Geometry: final body of the model. Coordinates: model frame, mm. Face numbers are marked on the shaded views. A direction names the side the tool comes from. Give positions to 0.01 mm unless a question says otherwise; leave off trailing zeros. Write each loop counter-clockwise with the first axis right and the second up, starting at its lowest first coordinate (ties: lowest second). Pieces come first, ordered by that corner, then holes. Notation, with made-up numbers: M -2,26.5 L 24,26.5 A29 ccw 24,49.5 Z; hole C -28,27 d7. An arc over 180 degrees is marked long. Use a Markdown table: item, result. Add a question column.
(1) Cut plane B-B (z = 21). Output: boundary loops of the cut face in (x, y).
(2) Draft query along Z for the marked faces 1, 2 and 3. Return one class per face: released by +Z, released by -Z, zero draft, split by the parting line, or undercut.
(3) Reachability of the marked faces 4 and 5 from +Z, -Z, +X, -X, +Y, -Y: full face, straight path, thin tool, end or side. Return the list, or none.
(4) Material intervals for L1, parallel to Z at x = 55.5, y = 70.5; L2, parallel to Z at x = 16.5, y = 74.5; L3, parallel to X at y = 66, z = 13.5, sorted ascending.
(5) Cut plane A-A (x = 50.5). Output: boundary loops of the cut face in (y, z).
(6) Pin query (flat end, axial travel): pin 1 Ø4 at (x, z) = (128.5, -13.5) entering from -Y; pin 2 Ø5 at (y, z) = (70, 12.5) entering from +X; pin 3 Ø1.6 at (y, z) = (72.5, -22) entering from -X; pin 4 Ø2 at (y, z) = (67.5, 26) entering from -X. Return the tip coordinate at first contact, or that it passes through.
```python
from build123d import *

# Parameters (mm, degrees)
BOX001002001_W                     = 70
BOX001002001_H                     = 15
BOX001002001_DEPTH                 = 2
BOX001002001002_W                  = 60
BOX001002001002_H                  = 15
BOX001002001002_DEPTH              = 2
BOX001002001002_PLACEMENT_ANGLE    = 209.99999
BOX001002001001_W                  = 60
BOX001002001001_H                  = 15
BOX001002001001_DEPTH              = 2
BOX001002001001_PITCH_ANGLE        = -31.999951
BOX001002001003_W                  = 26
BOX001002001003_H                  = 15
BOX001002001003_DEPTH              = 2
BOX001002001003_PLACEMENT_ANGLE    = 60.000023
BOX001002001003001_W               = 26
BOX001002001003001_H               = 15
BOX001002001003001_DEPTH           = 2
BOX001002001003001_PLACEMENT_ANGLE = 119.999977
BOX001002_W                        = 145
BOX001002_H                        = 15
BOX001002_DEPTH                    = 2


with BuildPart() as box001002001:
    # Box001002001 → Box001002001 (new body)
    with BuildSketch(Plane(origin=(49, -20, -23), x_dir=(1, 0, 0), z_dir=(0, 0, 1))):
        with Locations((35, 7.5)):
            Rectangle(BOX001002001_W, BOX001002001_H)
    extrude(amount=BOX001002001_DEPTH)


with BuildPart() as box001002001002:
    # Box001002001002 → Box001002001002 (new body)
    with BuildSketch(Plane.XY):
        with Locations((30, 7.5)):
            Rectangle(BOX001002001002_W, BOX001002001002_H)
    extrude(amount=BOX001002001002_DEPTH)


with BuildPart() as box001002001002_1:
    # Box001002001002 placement: moved
    add(box001002001002.part.moved(Location((49, -20, -21))).rotate(Axis((49, -20, -21), (0, 1, 0)), BOX001002001002_PLACEMENT_ANGLE))


with BuildPart() as box001002001001:
    # Box001002001001 → Box001002001001 (new body)
    with BuildSketch(Plane.XY):
        with Locations((30, 7.5)):
            Rectangle(BOX001002001001_W, BOX001002001001_H)
    extrude(amount=BOX001002001001_DEPTH)


with BuildPart() as box001002001001_1:
    # Box001002001001 pitch: moved
    add(box001002001001.part.rotate(Axis((0, 0, 0), (0, 1, 0)), BOX001002001001_PITCH_ANGLE))


with BuildPart() as box001002001001_2:
    # Box001002001001 placement: moved
    add(box001002001001_1.part.moved(Location((119, -20, -23))))


with BuildPart() as box001002001003:
    # Box001002001003 → Box001002001003 (new body)
    with BuildSketch(Plane.XY):
        with Locations((13, 7.5)):
            Rectangle(BOX001002001003_W, BOX001002001003_H)
    extrude(amount=BOX001002001003_DEPTH)


with BuildPart() as box001002001003_1:
    # Box001002001003 placement: moved
    add(box001002001003.part.moved(Location((-2, -20, 8))).rotate(Axis((-2, -20, 8), (0, -1, 0)), BOX001002001003_PLACEMENT_ANGLE))


with BuildPart() as box001002001003001:
    # Box001002001003001 → Box001002001003001 (new body)
    with BuildSketch(Plane.XY):
        with Locations((13, 7.5)):
            Rectangle(BOX001002001003001_W, BOX001002001003001_H)
    extrude(amount=BOX001002001003001_DEPTH)


with BuildPart() as box001002001003001_1:
    # Box001002001003001 placement: moved
    add(box001002001003001.part.moved(Location((169, -20, 9))).rotate(Axis((169, -20, 9), (0, -1, 0)), BOX001002001003001_PLACEMENT_ANGLE))


with BuildPart() as obj1:
    # Box001002 → Box001002 (new body)
    with BuildSketch(Plane(origin=(10, -20, 30), x_dir=(1, 0, 0), z_dir=(0, 0, 1))):
        with Locations((72.5, 7.5)):
            Rectangle(BOX001002_W, BOX001002_H)
    extrude(amount=BOX001002_DEPTH)

    # Fusion002001002001: union Box001002001, Box001002001002, Box001002001001, Box001002001003, Box001002001003001
    add(box001002001.part)
    add(box001002001002_1.part)
    add(box001002001001_2.part)
    add(box001002001003_1.part)
    add(box001002001003001_1.part)


with BuildPart() as obj1_1:
    # Fusion002001002001 placement: moved
    add(obj1.part.moved(Location((0, 85, 0))))


solid = obj1_1.part
```
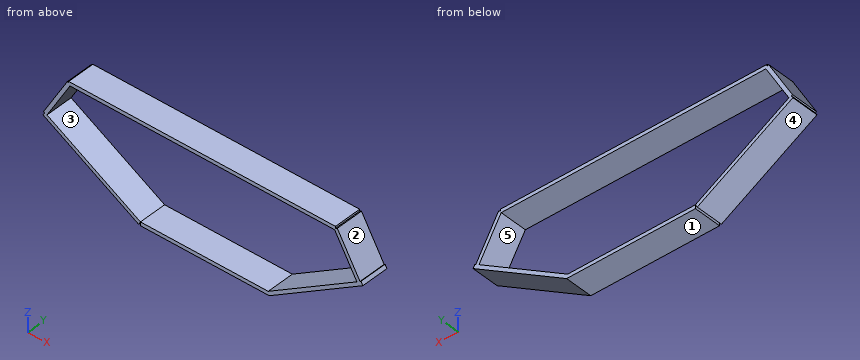
Answer list:
| question | item | result |
|---|---|---|
| 1 | outline | M 3.2,65 L 5.51,65 L 5.51,80 L 3.2,80 Z; M 159.76,65 L 162.07,65 L 162.07,80 L 159.76,80 Z |
| 2 | face 1 | released by -Z |
| 2 | face 2 | released by +Z |
| 2 | face 3 | undercut |
| 3 | face 4 | -Z, -X, +Y, -Y |
| 3 | face 5 | +Y, -Y |
| 4 | L1 | -23 to -21, 30 to 32 |
| 4 | L2 | -4.55 to -2.24, 30 to 32 |
| 4 | L3 | -1.13 to 1.18, 164.09 to 166.4 |
| 5 | outline | M 65,-23 L 80,-23 L 80,-21 L 65,-21 Z; M 65,30 L 80,30 L 80,32 L 65,32 Z |
| 6 | pin 1 | y = 65 |
| 6 | pin 2 | x = 169.13 |
| 6 | pin 3 | x = 45.35 |
| 6 | pin 4 | x = 5.51 |
